from build123d import *

# Parameters (mm, degrees)
SKETCH_2_W                                 = 125.5
SKETCH_2_H                                 = 80
EXTRUDE_1_DEPTH                            = 10.25
SKETCH_3_W                                 = 75
SKETCH_3_H                                 = 30
CUT_EXTRUDE_1_DEPTH                        = 15
SKETCH_4_R                                 = 2.5
EXTRUDE_2_DEPTH                            = 16
MIRROR_1_AT_THE_SECOND_PLANE_COPY_1_SKET_R = 2.5
MIRROR_1_AT_THE_SECOND_PLANE_COPY_1_DEPTH  = 16
SKETCH_5_W                                 = 108
SKETCH_5_H                                 = 10
CUT_EXTRUDE_2_DEPTH                        = 2


with BuildPart() as part:
    # 草图2 → 凸台-拉伸1 (new, symmetric)
    with BuildSketch(Plane(origin=(0, 0, 0), x_dir=(1, 0, 0), z_dir=(0, 1, 0))):
        Rectangle(SKETCH_2_W, SKETCH_2_H)
    extrude(amount=EXTRUDE_1_DEPTH, both=True)

    # 草图3 → 切除-拉伸1 (cut)
    with BuildSketch(Plane(origin=(0, 10.25, 0), x_dir=(1, 0, 0), z_dir=(0, 1, 0))):
        Rectangle(SKETCH_3_W, SKETCH_3_H)
    extrude(amount=-CUT_EXTRUDE_1_DEPTH, mode=Mode.SUBTRACT)

    # 草图4 → 凸台-拉伸2 (add)
    with BuildSketch(Plane.XZ.offset(10.25)):
        with Locations(Location((59.25, 36.5, 0), (0, 0, 270))):
            Circle(SKETCH_4_R)
    extrude_2 = extrude(amount=EXTRUDE_2_DEPTH)

    # 镜向1: 凸台-拉伸2 across plane
    add(extrude_2.mirror(Plane(origin=(0, 0, 0), x_dir=(0, 0, 1), z_dir=(1, 0, 0))))

    # 镜向1 at the second plane: 凸台-拉伸2 across plane
    add(extrude_2.mirror(Plane.XY))

    # 镜向1 at the second plane copy 1 sket → 镜向1 at the second plane copy 1 (add)
    with BuildSketch(Plane(origin=(0, -10.25, 0), x_dir=(-1, 0, 0), z_dir=(0, -1, 0))):
        with Locations(Location((59.25, 36.5, 0), (0, 0, 270))):
            Circle(MIRROR_1_AT_THE_SECOND_PLANE_COPY_1_SKET_R)
    extrude(amount=MIRROR_1_AT_THE_SECOND_PLANE_COPY_1_DEPTH)

    # 草图5 → 切除-拉伸2 (cut)
    with BuildSketch(Plane.XY.offset(40)):
        Rectangle(SKETCH_5_W, SKETCH_5_H)
    cut_extrude_2 = extrude(amount=-CUT_EXTRUDE_2_DEPTH, mode=Mode.SUBTRACT)

    # 镜向2: 切除-拉伸2 across plane
    add(cut_extrude_2.mirror(Plane.XY), mode=Mode.SUBTRACT)


solid = part.part
The listing builds one solid part. Answer for the finished solid, in the listing's coordinates (mm). A direction names the side the tool comes from. Round coordinates to 2 decimals unless told otherwise and drop trailing zeros. Write each loop counter-clockwise with the first axis right and the second up, starting at its lowest first coordinate (ties: lowest second). Pieces come first, ordered by that corner, then holes. Notation, with made-up numbers: (-33, 89.5) - (8, 89.5) arc R26 cw to (8, 128.5) - close; hole circle Ø10 at (2, 78). An arc over 180 degrees is marked (long way). Use a Markdown table: item, result. Add a question column.
1. The part is cut by section A-A (y = -2). Write down the section's boundary in (x, z).
2. The part is cut by section B-B (x = 59.25). Write down the section's boundary in (y, z).
3. Consider line 1 (X direction, y = -4, z = -12); line 2 (Z direction, x = 33, y = 5.5); line 3 (Z direction, x = -23, y = 4.5). Determine where each line is inside the solid, lowest interval first.
4. For a pull along X with two mould halves and no side action, classify faces 6 (the face through (-62.75, 0, 1)), 7 (the face through (62.75, 0, 1)), 8 (the face through (-1, 3, -15)), 9 (the face through (-59, -26.25, 37)) as +X half, -X half, draft (parallel to the pull), parting line (faces both ways), or undercut.
5. The part is cut by section C-C (z = 36.5). Write down the section's boundary in (x, y), and give its area (3 significant figures).
6. A tool of negligible diameter and unlimited length cuts with its end or side. For faces 1 (the face through (37.5, 3, 0)), 2 (the face through (59, -26.25, 37)), 3 (the face through (-1, 0, -38)), 4 (the face through (-1, 0, 38)), 5 (the face through (-58.29, -18.14, -34.19)), from which of +Z, -Z, +X, -X, +Y, -Y can it reach the whole face along a straight path? Write none if from no direction.
7. Flat-ended cylindrical pins translate along their axes: P1, Ø2, axis at x = -11, z = -39, coming from the -Y side; P2, Ø1.5, axis at x = -4.5, y = 3.5, coming from the +Z side; P3, Ø7.5, axis at x = -14.5, y = 3, coming from the -Z side; P4, Ø6, axis at x = 1, z = -6.5, coming from the +Y side. Find the tip coordinate at first contact, or state that the pin passes through.
8. The part is cut by section D-D (y = -17.5). Write down the section's boundary in (x, z), and give its area (3 significant figures).
Reported:
| question | item | result |
|---|---|---|
| 1 | outline | (-62.75, -40) - (-54, -40) - (-54, -38) - (54, -38) - (54, -40) - (62.75, -40) - (62.75, 40) - (54, 40) - (54, 38) - (-54, 38) - (-54, 40) - (-62.75, 40) - close; hole (-37.5, -15) - (37.5, -15) - (37.5, 15) - (-37.5, 15) - close |
| 2 | outline | (-26.25, -39) - (-10.25, -39) - (-10.25, -40) - (10.25, -40) - (10.25, 40) - (-10.25, 40) - (-10.25, 39) - (-26.25, 39) - (-26.25, 34) - (-10.25, 34) - (-10.25, -34) - (-26.25, -34) - close |
| 3 | line 1 | -62.75 to -37.5, 37.5 to 62.75 |
| 3 | line 2 | -40 to -15, 15 to 40 |
| 3 | line 3 | -38 to -15, 15 to 38 |
| 4 | face 6 | -X half |
| 4 | face 7 | +X half |
| 4 | face 8 | undercut |
| 4 | face 9 | draft |
| 5 | outline | (-62.75, -10.25) - (-61.75, -10.25) - (-61.75, -26.25) - (-56.75, -26.25) - (-56.75, -10.25) - (56.75, -10.25) - (56.75, -26.25) - (61.75, -26.25) - (61.75, -10.25) - (62.75, -10.25) - (62.75, 10.25) - (-62.75, 10.25) - close |
| 5 | area | 2,730 mm^2 |
| 6 | face 1 | +Y |
| 6 | face 2 | +Z, -Z, +X, -X, -Y |
| 6 | face 3 | -Z |
| 6 | face 4 | +Z |
| 6 | face 5 | -Y |
| 7 | P1 | y = -10.25 |
| 7 | P2 | z = 38 |
| 7 | P3 | z = -40 |
| 7 | P4 | y = -4.75 |
| 8 | outline | circle Ø5 at (-59.25, -36.5); circle Ø5 at (-59.25, 36.5); circle Ø5 at (59.25, -36.5); circle Ø5 at (59.25, 36.5) |
| 8 | area | 78.5 mm^2 |
